Read the model definition and answer for the solid it produces. Units are mm, in the model's axes. A direction names the side the tool comes from. Coordinates: 2 decimals unless noted, no trailing zeros. Write each loop counter-clockwise with the first axis right and the second up, starting at its lowest first coordinate (ties: lowest second). Pieces come first, ordered by that corner, then holes. Notation, with made-up numbers: (11.25, 57.25) - (51.25, 57.25) arc R21 ccw to (51.25, 78.25) - close; hole circle Ø7 at (20, -33). An arc over 180 degrees is marked (long way). Return JSON: item names as keys, results as strings.
Autodesk Inventor part; units mm, degrees
ref_plane "YZ Plane" through (0, 0, 0) normal (1, 0, 0) x (0, 1, 0)
ref_plane "XZ Plane" through (0, 0, 0) normal (0, 1, 0) x (-1, 0, 0)
ref_plane "XY Plane" through (0, 0, 0) normal (0, 0, 1) x (1, 0, 0)
sketch "Sketch1" plane through (0, 0, 0) normal (0, 0, 1) x (1, 0, 0)
  arc A0 (-28.9184, -1.6435) -> (-32.3684, 5.7551) centre (-35.052, 0) ccw
  line L0 (-28.702, 47.5942) -> (-28.702, -124.4009) construction
  line L1 (-32.3684, 5.7551) -> (-88.9, 32.1162)
  line L2 (-28.9184, -1.6435) -> (-86.2301, -215.5338)
  line L3 (-46.4564, 12.3244) -> (-66.802, 12.3244)
  line L4 (-60.4508, -95.6256) -> (-54.1008, -95.6256)
  line L5 (-73.152, -5.9838) -> (-73.152, -131.1779)
  line L6 (-73.152, -131.1779) -> (-63.627, -131.1779)
  line L7 (58.5667, 38.1) -> (-194.088, 38.1) construction
  line L8 (-95.25, 6.7162) -> (-95.25, -5.9838)
  line L9 (-95.25, 6.7162) -> (-88.9, 6.7162)
  line L10 (-88.9, 6.7162) -> (-88.9, 32.1162)
  line L11 (-95.25, -5.9838) -> (-73.152, -5.9838)
  line L12 (-95.25, -5.9838) -> (-95.25, -18.6838)
  line L13 (-95.25, -18.6838) -> (-89.3064, -18.6838)
  line L14 (-89.3064, -18.6838) -> (-89.3064, -24.6274)
  line L15 (-89.3064, -24.6274) -> (-95.25, -24.6274)
  line L16 (-95.25, -24.6274) -> (-95.25, -82.1838)
  line L17 (-95.25, -82.1838) -> (-82.55, -82.1838)
  line L18 (-89.3064, -18.6838) -> (-82.55, -18.6838)
  line L19 (-82.55, -18.6838) -> (-82.55, -82.1838)
  line L20 (-95.25, -82.1838) -> (-101.6, -82.1838)
  line L21 (-66.802, 12.3244) -> (-66.802, -31.3838)
  line L22 (-66.802, -31.3838) -> (-60.4508, -95.6256)
  line L23 (-82.55, -178.1009) -> (-76.2, -178.1009)
  line L24 (-82.55, -82.1838) -> (-82.55, -178.1009)
  line L25 (-86.2301, -215.5338) -> (-89.4051, -215.5338)
  line L26 (-89.4051, -215.5338) -> (-101.6, -82.1838)
  line L27 (-69.977, -5.9838) -> (-69.977, -31.3838)
  line L28 (-69.977, -31.3838) -> (-73.152, -31.3838)
  line L29 (-69.977, -5.9838) -> (-66.802, -5.9838)
  line L30 (-101.6, -82.1838) -> (-28.702, -82.1838) construction
  line L31 (0, -210.5351) -> (0, 86.485) construction
  point P0 (0, 0)
  dimension "d0" = 12.7
  dimension "d1" = 28.702
  dimension "d3" = 15
  dimension "d4" = 6.35
  dimension "d9" = 38.1
  dimension "d11" = 12.7
  dimension "d13" = 95.25
  dimension "d14" = 6.35
  dimension "d15" = 25.4
  dimension "d17" = 12.7
  dimension "d18" = 5.9436
  dimension "d19" = 5.9436
  dimension "d20" = 12.7
  dimension "d22" = 107.95
  dimension "d23" = 63.5
  dimension "d25" = 25.4
  dimension "d26" = 6.35
  dimension "d27" = 133.35
  dimension "d28" = 3.175
  dimension "d29" = 101.6
  dimension "d30" = 6.35
  dimension "d31" = 25
  dimension "d32" = 44.45
  dimension "d33" = 3.175
  dimension "d34" = 20.3456
  dimension "d35" = 9.525
revolve "Revolution1" add sketch "Sketch1" angle 360 about axis through (0, -210.5351, 0) along (0, 1, 0) contours L2 L23 L24 L19 L18 L13 L12 L11 L5 L6
properties part number "aluminum_carrier" material "Aluminum 6061"
(1) Which of the six approach directions +Z, -Z, +X, -X, +Y, -Y give full straight-line access (tool end or side, diameter ignored) to faces 4 (the face through (22, -131.178, 60)), 5 (the face through (22, -5.984, -70)), 6 (the face through (29, -18.684, 78))?
Answer:
{"face 4": "+Y", "face 5": "+Z, -Z, +X, -X, +Y", "face 6": "-Y"}
(2) Straight lines are drawn through the part: line 1 (Z direction, x = 0.5, y = -42.5); line 2 (Z direction, x = -37.5, y = -148.5); line 3 (X direction, y = -87, z = 21.5). For each, find the intervals that lie inside material, in ascending order. Write a range as from..to.
Answer:
{"line 1": "-82.55..-73.15, 73.15..82.55", "line 2": "-73.54..-57.05, 57.05..73.54", "line 3": "-79.7..-69.92, 69.92..79.7"}
(3) A cutting plane is placed at B-B (x = 0). Determine the outline of the cut face in (y, z).
Answer:
{"outline": "(-178.1, -82.55) - (-18.68, -82.55) - (-18.68, -95.25) - (-5.98, -95.25) - (-5.98, -73.15) - (-131.18, -73.15) - (-131.18, -63.63) - (-178.1, -76.2) - close; (-178.1, 76.2) - (-131.18, 63.63) - (-131.18, 73.15) - (-5.98, 73.15) - (-5.98, 95.25) - (-18.68, 95.25) - (-18.68, 82.55) - (-178.1, 82.55) - close"}
(4) Determine the mould class of faces 1 (the face through (75.587, -12.423, 57.958)), 2 (the face through (-24, -178.101, -73)), 3 (the face through (15.86, -69.46, 71.41)) for opening direction X: +X half, -X half, draft (parallel to the pull), parting line (faces both ways), or undercut.
Answer:
{"face 1": "parting line", "face 2": "draft", "face 3": "undercut"}
(5) Flat-ended cylindrical pins translate along their axes: P1, Ø1.5, axis at x = 13, y = -57.5, coming from the -Z side; P2, Ø1, axis at x = -40, y = -78, coming from the +Z side; P3, Ø1, axis at x = 25, y = -87.5, coming from the +Z side. Find the tip coordinate at first contact, or state that the pin passes through.
Answer:
{"P1": "z = -81.64", "P2": "z = 72.49", "P3": "z = 78.83"}
(6) A cutting plane is placed at A-A (z = 0). Determine the outline of the cut face in (x, y).
Answer:
{"outline": "(-95.25, -18.68) - (-82.55, -18.68) - (-82.55, -178.1) - (-76.2, -178.1) - (-63.63, -131.18) - (-73.15, -131.18) - (-73.15, -5.98) - (-95.25, -5.98) - close; (63.63, -131.18) - (76.2, -178.1) - (82.55, -178.1) - (82.55, -18.68) - (95.25, -18.68) - (95.25, -5.98) - (73.15, -5.98) - (73.15, -131.18) - close"}
(7) A cutting plane is placed at C-C (y = -46). Determine the outline of the cut face in (x, z), and give its area (3 significant figures).
Answer:
{"outline": "circle Ø165.1 at (0, 0); hole circle Ø146.3 at (0, 0)", "area": "4,600 mm²"}
